Geometry: final body of the model. Coordinates: model frame, mm. A direction names the side the tool comes from. Give positions to 0.01 mm unless a question says otherwise; leave off trailing zeros. Write each loop counter-clockwise with the first axis right and the second up, starting at its lowest first coordinate (ties: lowest second). Pieces come first, ordered by that corner, then holes.
Q1. Section C-C (y = -1.05). Return the cut outline in (x, z), plus the area to 3 significant figures.
Q2. Line query: line 1 (Z direction, x = -23, y = -0.5); line 2 (X direction, y = 1.6, z = 3.5); line 3 (Z direction, x = -19.5, y = 1.4). Output: solid intervals per line, ascending.
Q3. Section B-B (x = -28). Return the cut outline in (y, z).
Q4. Pin query (flat end, axial travel): pin 1 Ø0.6 at (x, y) = (-14.5, -0.5) entering from -Z; pin 2 Ø0.6 at (x, y) = (22, -1) entering from +Z; pin 3 Ø20 at (x, z) = (-0.5, 10) entering from -Y. Return the tip coordinate at first contact, or that it passes through.
Q5. Mould query, pull axis X, two halves, no side actions, for faces 4 (the flat face through (-1, 1, -20.75)), 5 (the flat face through (-1, 0, -23)), 6 (the cylindrical face through (48.7, -0.99, -31.28)). Classes: +X half, -X half, draft (parallel to the pull), parting line (faces both ways), or undercut.
Q6. Section D-D (z = -22). Return the cut outline in (x, y).
Q7. Section A-A (z = 19.5). Return the cut outline in (x, y).
Q8. Reachability of faces 1 (the flat face through (-49.5, 1, 0)), 2 (the cylindrical face through (-48.7, -0.99, 31.28)), 3 (the flat face through (1, -1, 31.55)) from +Z, -Z, +X, -X, +Y, -Y: full face, straight path, thin tool, end or side. Return the list, or none.
Autodesk Fusion 360 part; units mm, degrees
sketch "Sketch1" plane through (0, 0, 0) normal (0, 1, 0) x (1, 0, 0)
  line L0 (-52.5, 33.75) -> (52.5, 33.75)
  line L1 (52.5, 33.75) -> (52.5, -33.75)
  line L2 (52.5, -33.75) -> (-52.5, -33.75)
  line L3 (-52.5, -33.75) -> (-52.5, 33.75)
  line L4 (-52.5, 33.75) -> (52.5, -33.75) construction
  dimension "d115" = 105
  dimension "d116" = 67.5
extrude "Extrude1" add sketch "Sketch1" along normal blind 2
fillet "Fillet1" radius 5 4 edges at (-52.5, 1, 33.75) (52.5, 1, 33.75) (52.5, 1, -33.75) (-52.5, 1, -33.75)
sketch "Sketch2" plane through (0, 2, 0) normal (0, 1, 0) x (-1, 0, 0)
  arc A0 (47.5, -33.75) -> (52.5, -28.75) centre (47.5, -28.75) ccw
  line L0 (52.5, -28.75) -> (52.5, 28.75)
  arc A1 (52.5, 28.75) -> (47.5, 33.75) centre (47.5, 28.75) ccw
  line L1 (47.5, 33.75) -> (-47.5, 33.75)
  arc A2 (-47.5, 33.75) -> (-52.5, 28.75) centre (-47.5, 28.75) ccw
  line L2 (-52.5, 28.75) -> (-52.5, -28.75)
  arc A3 (-52.5, -28.75) -> (-47.5, -33.75) centre (-47.5, -28.75) ccw
  line L3 (-47.5, -33.75) -> (47.5, -33.75)
  line L4 (49.5, -20.75) -> (-49.5, -20.75)
  line L5 (-49.5, -20.75) -> (-49.5, 20.75)
  line L6 (-49.5, 20.75) -> (49.5, 20.75)
  line L7 (49.5, 20.75) -> (49.5, -20.75)
  line L8 (49.5, -20.75) -> (-49.5, 20.75) construction
  dimension "d120" = 99
  dimension "d121" = 41.5
extrude "Extrude2" cut sketch "Sketch2" against normal blind 2 contours L4 L5 L6 L7
sketch "Sketch3" plane through (0, 0, 0) normal (0, -1, 0) x (1, 0, 0)
  line L0 (49.5, 20.75) -> (49.5, -20.75)
  line L1 (49.5, -20.75) -> (-49.5, -20.75)
  line L2 (-49.5, -20.75) -> (-49.5, 20.75)
  line L3 (-49.5, 20.75) -> (49.5, 20.75)
  arc A0 (-52.5, -28.75) -> (-47.5, -33.75) centre (-47.5, -28.75) ccw
  line L4 (-47.5, -33.75) -> (47.5, -33.75)
  arc A1 (47.5, -33.75) -> (52.5, -28.75) centre (47.5, -28.75) ccw
  line L5 (52.5, -28.75) -> (52.5, 28.75)
  arc A2 (52.5, 28.75) -> (47.5, 33.75) centre (47.5, 28.75) ccw
  line L6 (47.5, 33.75) -> (-47.5, 33.75)
  arc A3 (-47.5, 33.75) -> (-52.5, 28.75) centre (-47.5, 28.75) ccw
  line L7 (-52.5, 28.75) -> (-52.5, -28.75)
  line L8 (-50.3, 28.75) -> (-50.3, -28.75)
  arc A4 (-50.3, -28.75) -> (-47.5, -31.55) centre (-47.5, -28.75) ccw
  line L9 (-47.5, -31.55) -> (47.5, -31.55)
  arc A5 (47.5, -31.55) -> (50.3, -28.75) centre (47.5, -28.75) ccw
  line L10 (50.3, -28.75) -> (50.3, 28.75)
  arc A6 (50.3, 28.75) -> (47.5, 31.55) centre (47.5, 28.75) ccw
  line L11 (47.5, 31.55) -> (-47.5, 31.55)
  arc A7 (-47.5, 31.55) -> (-50.3, 28.75) centre (-47.5, 28.75) ccw
  line L12 (-49.6448, 30.55) -> (49.6448, 30.55)
  line L13 (-49.6448, -30.55) -> (49.6448, -30.55)
  dimension "d124" = -2.2
  dimension "d125" = 1
  dimension "d126" = 1
extrude "Extrude3" add sketch "Sketch3" along normal blind 2 contours A6 L11 A7 L12 | A4 L9 A5 L13
Computed:
1. outline: (-49.64, -30.55) arc R2.8 ccw to (-47.5, -31.55) - (47.5, -31.55) arc R2.8 ccw to (49.64, -30.55) - close; (-49.64, 30.55) - (49.64, 30.55) arc R2.8 ccw to (47.5, 31.55) - (-47.5, 31.55) arc R2.8 ccw to start
1. area: 196 mm2
2. line 1: z = -31.55 to -30.55, 30.55 to 31.55
2. line 2: x = -52.5 to -49.5, 49.5 to 52.5
2. line 3: z = -33.75 to -20.75, 20.75 to 33.75
3. outline: (-2, -31.55) - (0, -31.55) - (0, -33.75) - (2, -33.75) - (2, -20.75) - (0, -20.75) - (0, -30.55) - (-2, -30.55) - close; (-2, 30.55) - (0, 30.55) - (0, 20.75) - (2, 20.75) - (2, 33.75) - (0, 33.75) - (0, 31.55) - (-2, 31.55) - close
4. pin 1: stops at z = -31.55
4. pin 2: stops at z = 31.55
4. pin 3: passes through
5. face 4: undercut
5. face 5: draft
5. face 6: +X half
6. outline: (-52.5, 0) - (52.5, 0) - (52.5, 2) - (-52.5, 2) - close
7. outline: (-52.5, 0) - (-49.5, 0) - (-49.5, 2) - (-52.5, 2) - close; (49.5, 0) - (52.5, 0) - (52.5, 2) - (49.5, 2) - close
8. face 1: +Y, -Y
8. face 2: +Z, -X, -Y
8. face 3: +Z, +X, -X, -Y
